Work out the finished part from the listing and answer in its coordinate system (mm). A direction names the side the tool comes from. Round coordinates to 2 decimals unless told otherwise and drop trailing zeros. Order: outer loops, then holes, each group sorted by start corner. A loop starts at its lowest first (then second) coordinate and runs counter-clockwise, first axis right, second up. Notation, with made-up numbers: M -19,40.25 L -5,40.25 A9 ccw -5,48.25 Z; hole C -15.5,54 d2. An arc over 180 degrees is marked long. Return JSON: item names as keys, results as strings.
from build123d import *

# Parameters (mm, degrees)
BOSS_EXTRUDE1_DEPTH                                 = 7.5
CBORE_FOR_M6_HEX_SOCKET_HEAD_CAP_SCREW1_D           = 6.4
CBORE_FOR_M6_HEX_SOCKET_HEAD_CAP_SCREW1_CBORE_D     = 11
CBORE_FOR_M6_HEX_SOCKET_HEAD_CAP_SCREW1_CBORE_DEPTH = 6.4
TAP_DRILL_FOR_M4_TAP1_D                             = 3.3
CBORE_FOR_M4_HEX_SOCKET_HEAD_CAP_SCREW1_D           = 4.5
CBORE_FOR_M4_HEX_SOCKET_HEAD_CAP_SCREW1_DEPTH       = 30
CBORE_FOR_M4_HEX_SOCKET_HEAD_CAP_SCREW1_CBORE_D     = 8
CBORE_FOR_M4_HEX_SOCKET_HEAD_CAP_SCREW1_CBORE_DEPTH = 16.4
FILLET1_R                                           = 1
CHAMFER1_SIZE                                       = 0.4


with BuildPart() as part:
    # Sketch1 → Boss-Extrude1 (new, symmetric)
    with BuildSketch(Plane.XY):
        Polygon((0, 0), (0, 16), (10, 16), (10, 6), (40, 6), (40, 0), (40, -14), (12, -14), align=None)
    extrude(amount=BOSS_EXTRUDE1_DEPTH, both=True)

    # CBORE for M6 Hex Socket Head Cap Screw1 (through all)
    with Locations(Plane(origin=(0, -14, 0), x_dir=(-1, 0, 0), z_dir=(0, -1, 0))):
        with Locations((-25, 0)):
            CounterBoreHole(CBORE_FOR_M6_HEX_SOCKET_HEAD_CAP_SCREW1_D / 2, CBORE_FOR_M6_HEX_SOCKET_HEAD_CAP_SCREW1_CBORE_D / 2, CBORE_FOR_M6_HEX_SOCKET_HEAD_CAP_SCREW1_CBORE_DEPTH)

    # Tap Drill for M4 Tap1 (through all)
    with Locations(Plane(origin=(16, 16, 0), x_dir=(0, 0, 1), z_dir=(0, 1, 0))):
        with Locations((0, -10)):
            Hole(TAP_DRILL_FOR_M4_TAP1_D / 2)

    # CBORE for M4 Hex Socket Head Cap Screw1
    with Locations(Plane(origin=(0, -14, 0), x_dir=(-1, 0, 0), z_dir=(0, -1, 0))):
        with Locations((-6, 0)):
            CounterBoreHole(CBORE_FOR_M4_HEX_SOCKET_HEAD_CAP_SCREW1_D / 2, CBORE_FOR_M4_HEX_SOCKET_HEAD_CAP_SCREW1_CBORE_D / 2, CBORE_FOR_M4_HEX_SOCKET_HEAD_CAP_SCREW1_CBORE_DEPTH, depth=CBORE_FOR_M4_HEX_SOCKET_HEAD_CAP_SCREW1_DEPTH)

    # Fillet1
    fillet1_edges = [part.edges().sort_by_distance(p)[0] for p in [
        (40, -4, -7.5),
        (40, -4, 7.5),
    ]]
    fillet(fillet1_edges, radius=FILLET1_R)

    # Chamfer1
    chamfer1_edges = [part.edges().sort_by_distance(p)[0] for p in [
        (25.5, -14, -7.5),
        (6, -7, -7.5),
        (0, 16, 0),
        (10, 16, 0),
        (10, 11, 7.5),
        (5, 16, 7.5),
        (0, 8, 7.5),
        (6, -7, 7.5),
        (40, 6, 0),
        (40, -14, 0),
        (24.5, 6, -7.5),
        (24.5, 6, 7.5),
        (39.707106781, 6, 7.207106781),
        (39.707106781, 6, -7.207106781),
        (39.707106781, -14, 7.207106781),
        (39.707106781, -14, -7.207106781),
        (0, 8, -7.5),
        (25.5, -14, 7.5),
        (5, 16, -7.5),
        (10, 11, -7.5),
    ]]
    chamfer(chamfer1_edges, length=CHAMFER1_SIZE)


solid = part.part
Item 1: Find section C-C (z = -1.75). Determine the outline of the cut face in (x, y), plus the area to 3 significant figures.
Output:
{"outline": "M 0,0 L 2.4,-2.8 L 2.4,2.4 L 4.59,2.4 L 4.59,16 L 0.4,16 L 0,15.6 Z; M 7.41,2.4 L 9.6,2.4 L 9.6,-11.2 L 12,-14 L 19.79,-14 L 19.79,-7.6 L 22.32,-7.6 L 22.32,6 L 10,6 L 10,15.6 L 9.6,16 L 7.41,16 Z; M 27.68,-7.6 L 30.21,-7.6 L 30.21,-14 L 39.6,-14 L 40,-13.6 L 40,5.6 L 39.6,6 L 27.68,6 Z", "area": "570 mm^2"}
Item 2: Which of the six approach directions +Z, -Z, +X, -X, +Y, -Y give full straight-line access (tool end or side, diameter ignored) to faces 1 (the flat face through (10, 11, 0)), 2 (the conical face through (39.542, 5.842, -7.03)), 3 (the flat face through (4, 2.4, 2))?
Output:
{"face 1": "+Z, -Z, +X, +Y", "face 2": "-Z, +X, +Y", "face 3": "-Y"}
Item 3: Find section A-A (x = 25). Determine the outline of the cut face in (y, z), plus the area to 3 significant figures.
Output:
{"outline": "M -14,-7.1 L -13.6,-7.5 L 5.6,-7.5 L 6,-7.1 L 6,-3.2 L -7.6,-3.2 L -7.6,-5.5 L -14,-5.5 Z; M -14,5.5 L -7.6,5.5 L -7.6,3.2 L 6,3.2 L 6,7.1 L 5.6,7.5 L -13.6,7.5 L -14,7.1 Z", "area": "142 mm^2"}
Item 4: Find section D-D (x = 17.5). Determine the outline of the cut face in (y, z), plus the area to 3 significant figures.
Output:
{"outline": "M -14,-7.1 L -13.6,-7.5 L 5.6,-7.5 L 6,-7.1 L 6,7.1 L 5.6,7.5 L -13.6,7.5 L -14,7.1 Z", "area": "300 mm^2"}
Item 5: Find section B-B (y = 1). Determine the outline of the cut face in (x, z), plus the area to 3 significant figures.
Output:
{"outline": "M 0,-7.1 L 0.4,-7.5 L 39,-7.5 A1 ccw 40,-6.5 L 40,6.5 A1 ccw 39,7.5 L 0.4,7.5 L 0,7.1 Z; hole C 6,0 d8; hole C 25,0 d6.4", "area": "517 mm^2"}
Item 6: Consider line 1 along Z through (x, y) = (6, 10); line 2 along Z through (x, y) = (6, -5.75); line 3 along X through (y, z) = (12.5, -4). Determine where each line is inside the solid, lowest interval first. Write a range as [from, to].
Output:
{"line 1": "z = [-7.5, -2.25], [2.25, 7.5]", "line 2": "z = [-7.5, -4], [4, 7.5]", "line 3": "x = [0, 10]"}
Item 7: Each of these flat-tipped pins is pushed along its axis until it touches: pin 1 (3 mm diameter, centred on x = 25.5, z = 3.5, fed in from -Y); pin 2 (9 mm diameter, centred on x = 6.5, z = -0.5, fed in from -Y); pin 3 (5 mm diameter, centred on y = -7.5, z = -3, fed in from -X). Where does it stop, or does it pass through?
Output:
{"pin 1": "stops at y = -7.6", "pin 2": "stops at y = -12.83", "pin 3": "stops at x = 4.36"}
Item 8: The mould has two halves that part along Z. Classify faces 4 (the flat face through (4, 16, 2)), 5 (the cylindrical face through (21.8, -0.7, -0.1)), 6 (the flat face through (20, -2, 7.5)): pulls with the +Z half, pulls with the -Z half, needs draft (parallel to the pull), parting line crosses it, or undercut.
Output:
{"face 4": "needs draft", "face 5": "undercut", "face 6": "pulls with the +Z half"}
